from build123d import *

# Parameters (mm, degrees)
BOSS_EXTRUDE1_DEPTH      = 3
SKETCH2_R                = 2.75
CUT_EXTRUDE1_DEPTH       = 4
SKETCH3_W                = 39.2
SKETCH3_H                = 3
BOSS_EXTRUDE2_DEPTH      = 42
SKETCH6_R                = 8
SKETCH6_R_2              = 1.75
CUT_EXTRUDE2_DEPTH       = 31.5
CUT_EXTRUDE2_DEPTH_BACK  = 34.5
SKETCH7_W                = 3
SKETCH7_H                = 42
BOSS_EXTRUDE3_DEPTH      = 30.5
BOSS_EXTRUDE3_DEPTH_BACK = 33.5
CUT_EXTRUDE5_DEPTH       = 77.4
CUT_EXTRUDE5_DEPTH_BACK  = 90.6
SKETCH9_R                = 4.75
SKETCH9_R_2              = 2.75
BOSS_EXTRUDE4_DEPTH      = 4.5


with BuildPart() as part:
    # Sketch1 → Boss-Extrude1 (new body)
    with BuildSketch(Plane(origin=(0, 0, 0), x_dir=(1, 0, 0), z_dir=(0, 1, 0))):
        with BuildLine():
            Line((78, 32), (-78, 32))
            ThreePointArc((-78, 32), (-81.535533906, 30.535533906), (-83, 27))
            Line((-83, 27), (-83, -27))
            ThreePointArc((-83, -27), (-81.535533906, -30.535533906), (-78, -32))
            Line((-78, -32), (78, -32))
            ThreePointArc((78, -32), (81.535533906, -30.535533906), (83, -27))
            Line((83, -27), (83, 27))
            ThreePointArc((83, 27), (81.535533906, 30.535533906), (78, 32))
        make_face()
    extrude(amount=BOSS_EXTRUDE1_DEPTH)

    # Sketch2 → Cut-Extrude1 (cut, through all)
    with BuildSketch(Plane(origin=(0, 3, 0), x_dir=(1, 0, 0), z_dir=(0, 1, 0))):
        with Locations((44, -15)):
            Circle(SKETCH2_R)
        with Locations((44, 15)):
            Circle(SKETCH2_R)
        with Locations((-18, 0)):
            Circle(SKETCH2_R)
    extrude(amount=-CUT_EXTRUDE1_DEPTH, mode=Mode.SUBTRACT)

    # Sketch3 → Boss-Extrude2 (add)
    with BuildSketch(Plane(origin=(0, 3, 0), x_dir=(1, 0, 0), z_dir=(0, 1, 0))):
        with Locations((13, 0)):
            Rectangle(SKETCH3_W, SKETCH3_H)
    extrude(amount=BOSS_EXTRUDE2_DEPTH)

    # Sketch6 → Cut-Extrude2 (cut, two sides)
    with BuildSketch(Plane(origin=(0, 0, -1.5), x_dir=(-1, 0, 0), z_dir=(0, 0, -1))) as cut_extrude2_sk:
        with Locations((-13, 24)):
            Circle(SKETCH6_R)
        with Locations((-4.161165235, 15.161165235)):
            Circle(SKETCH6_R_2)
        with Locations((-21.838834765, 15.161165235)):
            Circle(SKETCH6_R_2)
        with Locations((-21.838834765, 32.838834765)):
            Circle(SKETCH6_R_2)
        with Locations((-4.161165235, 32.838834765)):
            Circle(SKETCH6_R_2)
    extrude(amount=CUT_EXTRUDE2_DEPTH, mode=Mode.SUBTRACT)
    extrude(cut_extrude2_sk.sketch, amount=-CUT_EXTRUDE2_DEPTH_BACK, mode=Mode.SUBTRACT)

    # Sketch7 → Boss-Extrude3 (add, two sides)
    with BuildSketch(Plane(origin=(0, 0, -1.5), x_dir=(-1, 0, 0), z_dir=(0, 0, -1))) as boss_extrude3_sk:
        with Locations((-31.1, 24)):
            Rectangle(SKETCH7_W, SKETCH7_H)
        with Locations((5.1, 24)):
            Rectangle(SKETCH7_W, SKETCH7_H)
    extrude(amount=BOSS_EXTRUDE3_DEPTH)
    extrude(boss_extrude3_sk.sketch, amount=-BOSS_EXTRUDE3_DEPTH_BACK)

    # Sketch8 → Cut-Extrude5 (cut, two sides)
    with BuildSketch(Plane.ZY.offset(6.6)) as cut_extrude5_sk:
        Polygon((-1.5, 45), (-32, 3), (-32, 45), align=None)
        Polygon((1.5, 45), (32, 3), (32, 45), align=None)
    extrude(amount=CUT_EXTRUDE5_DEPTH, mode=Mode.SUBTRACT)
    extrude(cut_extrude5_sk.sketch, amount=-CUT_EXTRUDE5_DEPTH_BACK, mode=Mode.SUBTRACT)

    # Sketch9 → Boss-Extrude4 (add)
    with BuildSketch(Plane.XZ):
        with Locations((-18, 0)):
            Circle(SKETCH9_R)
        with Locations((-18, 0)):
            Circle(SKETCH9_R_2, mode=Mode.SUBTRACT)
        with Locations((44, -15)):
            Circle(SKETCH9_R)
        with Locations((44, -15)):
            Circle(SKETCH9_R_2, mode=Mode.SUBTRACT)
        with Locations((44, 15)):
            Circle(SKETCH9_R)
        with Locations((44, 15)):
            Circle(SKETCH9_R_2, mode=Mode.SUBTRACT)
    extrude(amount=BOSS_EXTRUDE4_DEPTH)


solid = part.part
CAD build for the part. Positions are in the model's coordinates, mm. A direction names the side the tool comes from. Give positions to 0.01 mm unless a question says otherwise; leave off trailing zeros. Write each loop counter-clockwise with the first axis right and the second up, starting at its lowest first coordinate (ties: lowest second). Pieces come first, ordered by that corner, then holes. Notation, with made-up numbers: (2.25, -13.5) - (53.25, -13.5) arc R21 cw to (53.25, 21.5) - close; hole circle Ø10 at (27, 2.5). An arc over 180 degrees is marked (long way). Answer as CSV lines item,"result".
Q1. Pull direction X, two halves, no side cores. Call faces 6 (the face through (23.13, 16.34, -0.02)), 7 (the face through (20, 19, -1.5)), 8 (the face through (81, 1, 31)), 9 (the face through (-1, 0, 0)): released by +X, released by -X, zero draft, split by the parting line, or undercut.
Result set:
face 6,"undercut"
face 7,"undercut"
face 8,"released by +X"
face 9,"zero draft"
Q2. Flat gauge pins, fed straight in: pin 1 Ø1 at (x, z) = (56.5, -4.5) entering from -Y; pin 2 Ø8 at (x, y) = (-7, 17.5) entering from -Z; pin 3 Ø5.5 at (x, y) = (21.84, 15.16) entering from -Z. Where does each tip first touch, or does it go through?
Result set:
pin 1,"y = 0"
pin 2,"z = -24.36"
pin 3,"z = -1.5"
Q3. Band-saw the part on D-D (x = -18). Give the cut face in (y, z), and give its area (4 significant figures).
Result set:
outline,"(-4.5, -4.75) - (0, -4.75) - (0, -32) - (3, -32) - (3, -2.75) - (-4.5, -2.75) - close; (-4.5, 2.75) - (3, 2.75) - (3, 32) - (0, 32) - (0, 4.75) - (-4.5, 4.75) - close"
area,"193.5 mm²"
Q4. Drill centre lines: line 1 (Z direction, x = 44, y = -1.05); line 2 (Z direction, x = 44, y = 2); line 3 (Z direction, x = -18, y = 1.5). Where is each one in solid material? Low to high. Write a range as from..to.
Result set:
line 1,"-19.75..-17.75, -12.25..-10.25, 10.25..12.25, 17.75..19.75"
line 2,"-32..-17.75, -12.25..12.25, 17.75..32"
line 3,"-32..-2.75, 2.75..32"
Q5. Band-saw the part on C-C (y = 24). Give the cut face in (x, z), and give its area (3 significant figures).
Result set:
outline,"(-6.6, -16.75) - (-3.6, -16.75) - (-3.6, -1.5) - (5, -1.5) - (5, 1.5) - (-3.6, 1.5) - (-3.6, 16.75) - (-6.6, 16.75) - close; (21, -1.5) - (29.6, -1.5) - (29.6, -16.75) - (32.6, -16.75) - (32.6, 16.75) - (29.6, 16.75) - (29.6, 1.5) - (21, 1.5) - close"
area,"253 mm²"
Q6. 3-axis set-ups, long thin cutter, end or side, ignore diameter. For faces 1 (the face through (-45, 3, 0)), 2 (the face through (32.6, 19, 0)), 3 (the face through (20, 19, 1.5)), 4 (the face through (47, -4.5, -15)), 5 (the face through (4.389, 16.896, -0.021)): which of +Z, -Z, +X, -X, +Y, -Y reach the whole face in a straight line?
Result set:
face 1,"+Z, -Z, -X, +Y"
face 2,"+Z, -Z, +X, +Y"
face 3,"+Z, +Y"
face 4,"+Z, -Z, +X, -X, -Y"
face 5,"+Z, -Z"
Q7. Band-saw the part on A-A (x = 44). Give the cut face in (y, z), and give its area (3 significant figures).
Result set:
outline,"(-4.5, -19.75) - (0, -19.75) - (0, -32) - (3, -32) - (3, -17.75) - (-4.5, -17.75) - close; (-4.5, -12.25) - (3, -12.25) - (3, 12.25) - (-4.5, 12.25) - (-4.5, 10.25) - (0, 10.25) - (0, -10.25) - (-4.5, -10.25) - close; (-4.5, 17.75) - (3, 17.75) - (3, 32) - (0, 32) - (0, 19.75) - (-4.5, 19.75) - close"
area,"195 mm²"
Q8. Band-saw the part on B-B (z = 0). Give the cut face in (x, y).
Result set:
outline,"(-83, 0) - (-22.75, 0) - (-22.75, -4.5) - (-20.75, -4.5) - (-20.75, 3) - (-83, 3) - close; (-15.25, -4.5) - (-13.25, -4.5) - (-13.25, 0) - (83, 0) - (83, 3) - (32.6, 3) - (32.6, 45) - (-6.6, 45) - (-6.6, 3) - (-15.25, 3) - close; hole circle Ø3.5 at (4.16, 15.16); hole circle Ø3.5 at (4.16, 32.84); hole circle Ø16 at (13, 24); hole circle Ø3.5 at (21.84, 15.16); hole circle Ø3.5 at (21.84, 32.84)"
